Model file for the job. Use its own axes, mm. Face numbers are marked on the shaded views. A direction names the side the tool comes from. Round coordinates to 2 decimals unless told otherwise and drop trailing zeros. Order: outer loops, then holes, each group sorted by start corner. A loop starts at its lowest first (then second) coordinate and runs counter-clockwise, first axis right, second up. Notation, with made-up numbers: (88, 55.25) -> (109, 55.25) arc R19 ccw to (109, 77.25) -> close; hole circle Ø7 at (41, -17). An arc over 180 degrees is marked (long way). Put each result on its own line as item: value. Start each with the question number.
Q1. Flat gauge pin, fed straight in: P1, Ø12, axis at x = -35, y = 29, coming from the +Z side. Where does the tip first touch, or does it go through?
Q2. 3-axis set-ups, long thin cutter, end or side, ignore diameter. For the marked faces 4 and 5: which of +Z, -Z, +X, -X, +Y, -Y reach the whole face in a straight line?
Q3. Cut at B-B, the plane y = 16. List the corners of the cut face in (x, z).
Q4. Cut at A-A, the plane z = 16. List the corners of the cut face in (x, y).
Q5. Pull direction Y, two halves, no side cores. Call the marked faces 1, 2 and 3: released by +Y, released by -Y, zero draft, split by the parting line, or undercut.
Q6. Cut at C-C, the plane x = 14.5. List the corners of the cut face in (y, z), and give its area (3 significant figures).
Q7. Probe L1, parallel to X at y = 8, z = 32.5; L2, parallel to Y at x = -36.5, z = 21.5; L3, parallel to Z at x = 8, y = -31. List the from-to ranges inside material, lowest first.
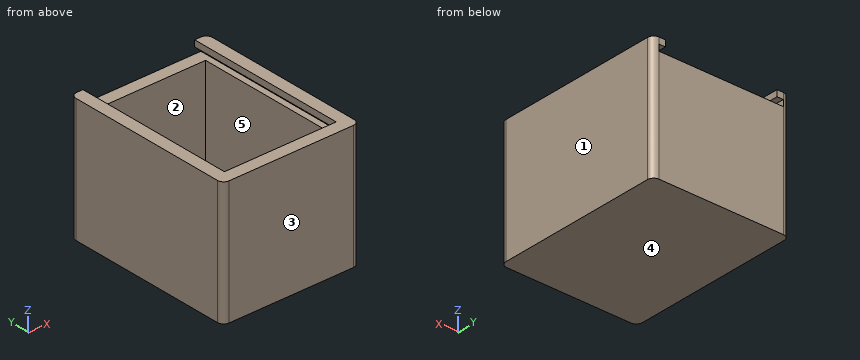
from build123d import *

# Parameters (mm, degrees)
F1_DEPTH  = 100
F2_W      = 90
F2_H      = 120
F3_DEPTH  = 90
F4_W      = 120
F4_H      = 5
F5_DEPTH  = 5
F6_W      = 120
F6_H      = 5
F7_DEPTH  = 5
F8_W      = 90
F8_H      = 10
F9_DEPTH  = 10
F10_W     = 10
F10_H     = 5
F11_DEPTH = 5
F12_W     = 10
F12_H     = 5
F13_DEPTH = 5


with BuildPart() as f1:
    # F0 (on Top) → F1 (new body)
    with BuildSketch(Plane.XY):
        with BuildLine():
            Line((-50, -70), (50, -70))
            ThreePointArc((50, -70), (53.535534, -68.535534), (55, -65))
            Line((55, -65), (55, 65))
            ThreePointArc((55, 65), (53.535534, 68.535534), (50, 70))
            Line((50, 70), (-50, 70))
            ThreePointArc((-50, 70), (-53.535534, 68.535534), (-55, 65))
            Line((-55, 65), (-55, -65))
            ThreePointArc((-55, -65), (-53.535534, -68.535534), (-50, -70))
        make_face()
    extrude(amount=F1_DEPTH)

    # F2 (on face) → F3 (cut)
    with BuildSketch(Plane.XY.offset(100)):
        Rectangle(F2_W, F2_H)
    extrude(amount=-F3_DEPTH, mode=Mode.SUBTRACT)

    # F4 (on face) → F5 (cut)
    with BuildSketch(Plane(origin=(45, 0, 0), x_dir=(0, -1, 0), z_dir=(-1, 0, 0))):
        with Locations((0, 92.5)):
            Rectangle(F4_W, F4_H)
    extrude(amount=-F5_DEPTH, mode=Mode.SUBTRACT)

    # F6 (on face) → F7 (cut)
    with BuildSketch(Plane.YZ.offset(-45)):
        with Locations((0, 92.5)):
            Rectangle(F6_W, F6_H)
    extrude(amount=-F7_DEPTH, mode=Mode.SUBTRACT)

    # F8 (on face) → F9 (cut)
    with BuildSketch(Plane.XZ.offset(-60)):
        with Locations((0, 95)):
            Rectangle(F8_W, F8_H)
    extrude(amount=-F9_DEPTH, mode=Mode.SUBTRACT)

    # F10 (on face) → F11 (cut)
    with BuildSketch(Plane(origin=(45, 0, 0), x_dir=(0, -1, 0), z_dir=(-1, 0, 0))):
        with Locations((-65, 92.5)):
            Rectangle(F10_W, F10_H)
    extrude(amount=-F11_DEPTH, mode=Mode.SUBTRACT)

    # F12 (on face) → F13 (cut)
    with BuildSketch(Plane.YZ.offset(-45)):
        with Locations((65, 92.5)):
            Rectangle(F12_W, F12_H)
    extrude(amount=-F13_DEPTH, mode=Mode.SUBTRACT)


solid = f1.part
Ans:
1. P1: stops at z = 10
2. face 4: -Z, +X, -X, +Y, -Y
2. face 5: +Z
3. outline: (-55, 0) -> (55, 0) -> (55, 100) -> (45, 100) -> (45, 95) -> (50, 95) -> (50, 90) -> (45, 90) -> (45, 10) -> (-45, 10) -> (-45, 90) -> (-50, 90) -> (-50, 95) -> (-45, 95) -> (-45, 100) -> (-55, 100) -> close
4. outline: (-55, -65) arc R5 ccw to (-50, -70) -> (50, -70) arc R5 ccw to (55, -65) -> (55, 65) arc R5 ccw to (50, 70) -> (-50, 70) arc R5 ccw to (-55, 65) -> close; hole (-45, -60) -> (45, -60) -> (45, 60) -> (-45, 60) -> close
5. face 1: zero draft
5. face 2: undercut
5. face 3: released by -Y
6. outline: (-70, 0) -> (70, 0) -> (70, 90) -> (60, 90) -> (60, 10) -> (-60, 10) -> (-60, 100) -> (-70, 100) -> close
6. area: 3,100 mm^2
7. L1: x = -55 to -45, 45 to 55
7. L2: y = -70 to -60, 60 to 70
7. L3: z = 0 to 10
